Here's how the part is built. I have some questions about the finished solid (model axes, mm). Coordinates: 2 decimals unless noted, no trailing zeros. Write each loop counter-clockwise with the first axis right and the second up, starting at its lowest first coordinate (ties: lowest second). Pieces come first, ordered by that corner, then holes. Notation, with made-up numbers: (24, -30.75) -> (28, -30.75) arc R37 ccw to (28, 8.25) -> close; hole circle Ø6 at (66.25, 72.5). An arc over 180 degrees is marked (long way). Put each result on its own line as item: value.
```python
from build123d import *

# Parameters (mm, degrees)
SKETCH_1_W          = 50
SKETCH_1_H          = 30
EXTRUDE_1_DEPTH     = 12
SKETCH_2_R          = 2
CUT_EXTRUDE_1_DEPTH = 12
FILLET_1_R          = 5


with BuildPart() as part:
    # 草图1 → 凸台-拉伸1 (new body)
    with BuildSketch(Plane.XY):
        with Locations((25, 15)):
            Rectangle(SKETCH_1_W, SKETCH_1_H)
    extrude(amount=-EXTRUDE_1_DEPTH)

    # 草图2 → 切除-拉伸1 (cut)
    with BuildSketch(Plane.XY):
        with Locations((44, 22)):
            Circle(SKETCH_2_R)
        with Locations(Location((44, 8, 0), (0, 0, 180))):
            Circle(SKETCH_2_R)
        with Locations((32, 22)):
            Circle(SKETCH_2_R)
        with Locations(Location((32, 8, 0), (0, 0, 180))):
            Circle(SKETCH_2_R)
    extrude(amount=-CUT_EXTRUDE_1_DEPTH, mode=Mode.SUBTRACT)

    # 圆角1
    fillet_1_edges = [part.edges().sort_by_distance(p)[0] for p in [
        (0, 30, -6),
        (50, 30, -6),
        (50, 0, -6),
        (0, 0, -6),
    ]]
    fillet(fillet_1_edges, radius=FILLET_1_R)


solid = part.part
```
Item 1: Imagine slicing it at B-B on y = 22. Write out the boundary of the cut face in (x, z), then the cut area to 3 significant figures.
Output:
outline: (0, -12) -> (30, -12) -> (30, 0) -> (0, 0) -> close; (34, -12) -> (42, -12) -> (42, 0) -> (34, 0) -> close; (46, -12) -> (50, -12) -> (50, 0) -> (46, 0) -> close
area: 504 mm²
Item 2: Please list where these lines run through material, in increasing order: line 1 along Y through (x, z) = (44, -9); line 2 along X through (y, z) = (8, -3.25); line 3 along X through (y, z) = (7.5, -9.5). Write a range as from..to.
Output:
line 1: y = 0..6, 10..20, 24..30
line 2: x = 0..30, 34..42, 46..50
line 3: x = 0..30.06, 33.94..42.06, 45.94..50
Item 3: Imagine slicing it at C-C on z = -10. Write out the boundary of the cut face in (x, y).
Output:
outline: (0, 5) arc R5 ccw to (5, 0) -> (45, 0) arc R5 ccw to (50, 5) -> (50, 25) arc R5 ccw to (45, 30) -> (5, 30) arc R5 ccw to (0, 25) -> close; hole circle Ø4 at (32, 8); hole circle Ø4 at (32, 22); hole circle Ø4 at (44, 8); hole circle Ø4 at (44, 22)
Item 4: If we mould it in two halves opening along Y, with no side actions, what happens to faces 1 (the flat face through (0, 15, -6)), 2 (the cylindrical face through (30.092, 7.399, -5.916)), 3 (the cylindrical face through (48, 1, -6))? For each: released by +Y, released by -Y, zero draft, split by the parting line, or undercut.
Output:
face 1: zero draft
face 2: undercut
face 3: released by -Y
Item 5: For P1, Ø3.5, axis at x = 44, y = 22, coming from the +Z side, with a flat end and sliding along its axis, tell me the tip position at first contact or that it passes through.
Output:
P1: passes through
Item 6: Imagine slicing it at D-D on x = 47. Write out the boundary of the cut face in (y, z), then the cut area to 3 significant figures.
Output:
outline: (0.42, -12) -> (29.58, -12) -> (29.58, 0) -> (0.42, 0) -> close
area: 350 mm²
Item 7: Imagine slicing it at A-A on x = 32. Write out the boundary of the cut face in (y, z).
Output:
outline: (0, -12) -> (6, -12) -> (6, 0) -> (0, 0) -> close; (10, -12) -> (20, -12) -> (20, 0) -> (10, 0) -> close; (24, -12) -> (30, -12) -> (30, 0) -> (24, 0) -> close
